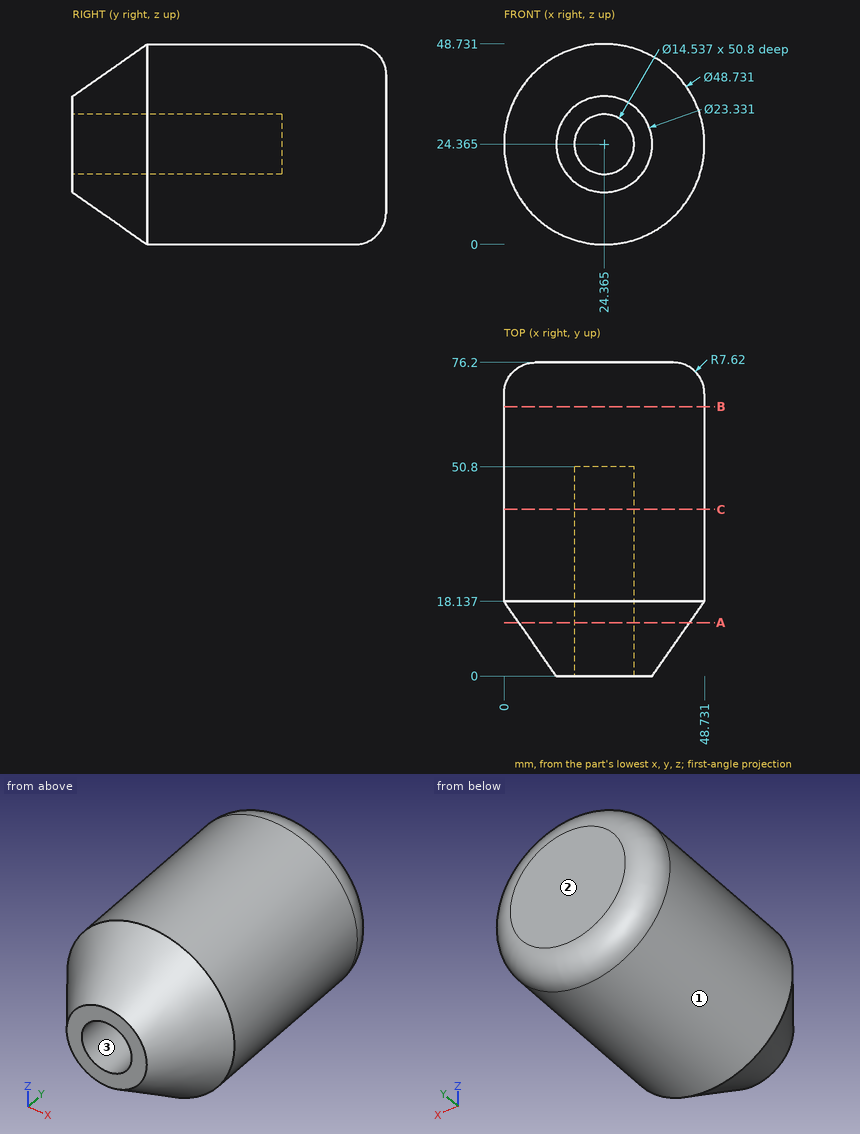
Verification items for this drawing (mm, ordinates from the low corner). Give positions to 0.01 mm unless a question says otherwise; leave off trailing zeros. Loops run counter-clockwise (first coordinate to the right, second up) from the corner with the lowest first, then second, coordinate; pieces in that order, holes last. Notation, with made-up numbers: M 84.5,-38.5 L 119.5,-38.5 A21 cw 119.5,-34.5 Z; hole C 78.5,13 d5. An arc over 180 degrees is marked long. Answer as CSV lines item,"result".
Item 1: Release check for a two-part mould opening along X. For the marked faces 1, 2 and 3 record: pulls with the +X half, pulls with the -X half, needs draft (parallel to the pull), parting line crosses it, or undercut.
Values:
face 1,"parting line crosses it"
face 2,"needs draft"
face 3,"undercut"
Item 2: Cross-section at C-C on y = 40.5. Record the cut outline in (x, z) (1 decimal).
Values:
outline,"C 24.4,24.4 d48.7; hole C 24.4,24.4 d14.5"
Item 3: Cross-section at A-A on y = 13. Record the cut outline in (x, z) (1 decimal).
Values:
outline,"C 24.4,24.4 d41.5; hole C 24.4,24.4 d14.5"
Item 4: Depth check by flat-ended pin: P1, Ø1.5, axis at y = 25, z = 15, coming from the -X side (1 decimal); P2, Ø4, axis at x = 15.5, y = 48, coming from the -Z side; P3, Ø10, axis at y = 18.5, z = 10, coming from the -X side. Enter the tip coordinate at first touch or a pass-through.
Values:
P1,"stops at x = 1.6"
P2,"stops at z = 0.99"
P3,"stops at x = 1.87"
Item 5: Cross-section at B-B on y = 65.5. Record the cut outline in (x, z) (1 decimal).
Values:
outline,"C 24.4,24.4 d48.7"
Item 6: Material ranges on line 1 (X direction, y = 40, z = 25) (1 decimal); line 2 (X direction, y = 7.5, z = 24) (1 decimal); line 3 (Z direction, x = 29, y = 66) (1 decimal), recorded low to high.
Values:
line 1,"x = 0 to 17.1, 31.6 to 48.7"
line 2,"x = 7.5 to 17.1, 31.6 to 41.3"
line 3,"z = 0.4 to 48.3"
